Check sheet for the modelled part. Datum: model origin and axes. Units: mm. A direction names the side the tool comes from. Round coordinates to 2 decimals unless told otherwise and drop trailing zeros. Write each loop counter-clockwise with the first axis right and the second up, starting at its lowest first coordinate (ties: lowest second). Pieces come first, ordered by that corner, then holes.
Autodesk Inventor part; units mm, degrees
ref_plane "YZ Plane" through (0, 0, 0) normal (1, 0, 0) x (0, 1, 0)
ref_plane "XZ Plane" through (0, 0, 0) normal (0, 1, 0) x (-1, 0, 0)
ref_plane "XY Plane" through (0, 0, 0) normal (0, 0, 1) x (1, 0, 0)
sketch "スケッチ1" plane through (0, 0, 0) normal (0, 0, 1) x (1, 0, 0)
  line L0 (-120.5, 11.775) -> (120.5, 11.775) construction
  line L1 (120.5, 11.775) -> (120.5, -11.775) construction
  line L2 (120.5, -11.775) -> (-120.5, -11.775) construction
  line L3 (-120.5, -11.775) -> (-120.5, 11.775) construction
  circle A0 centre (-120.5, -11.775) radius 2.25
  circle A1 centre (-120.5, 11.775) radius 2.25
  circle A2 centre (-36.5, -11.775) radius 2.25
  circle A3 centre (42.5, -11.775) radius 2.25
  circle A4 centre (120.5, -11.775) radius 2.25
  line L4 (-129.5, 22.275) -> (-129.5, -20.275) construction
  line L5 (-129.5, 22.275) -> (129.5, 22.275) construction
  line L6 (129.5, 22.275) -> (129.5, -20.275) construction
  line L7 (129.5, -20.275) -> (-129.5, -20.275) construction
  circle A5 centre (-42.5, 17.275) radius 2.25
  circle A6 centre (42.5, 17.275) radius 2.25
  circle A7 centre (120.5, 11.775) radius 2.25
  line L8 (-129.5, -20.275) -> (129.5, -20.275)
  line L9 (129.5, -20.275) -> (129.5, 27.275)
  line L10 (129.5, 27.275) -> (-129.5, 27.275)
  line L11 (-129.5, 27.275) -> (-129.5, -20.275)
  point P0 (0, 0)
  point P1 (-120.5, 0)
  point P2 (0, 11.775)
  dimension "d0" = 23.55
  dimension "d1" = 84
  dimension "d3" = 79
  dimension "d4" = 78
  dimension "d5" = 4.5
  dimension "d6" = 9
  dimension "d7" = 9
  dimension "d8" = 8.5
  dimension "d9" = 10.5
  dimension "d10" = 5.5
  dimension "d11" = 78.1937
  dimension "d12" = 78.1937
  dimension "d13" = 78
  dimension "d14" = 85
  dimension "d15" = 78
  dimension "d16" = 5
extrude "押し出し1" add sketch "スケッチ1" along normal blind 4
sketch "スケッチ2" plane through (0, 0, 0) normal (0, 0, -1) x (-1, 0, 0)
  line L0 (129.5, 22.275) -> (-129.5, 22.275) construction
  line L1 (-129.5, 22.275) -> (129.5, 22.275)
  line L2 (129.5, 22.275) -> (129.5, 27.275)
  line L3 (129.5, 27.275) -> (-129.5, 27.275)
  line L4 (-129.5, 27.275) -> (-129.5, 22.275)
  line L5 (-129.5, 27.275) -> (129.5, 27.275) construction
  point P0 (0, 0)
extrude "押し出し2" add sketch "スケッチ2" along normal blind 47.4
fillet "フィレット1" radius 4 2 edges at (-129.5, -20.275, 2) (129.5, -20.275, 2)
fillet "フィレット2" [suppressed]
fillet "フィレット3" radius 4 2 edges at (129.5, 27.275, -21.7) (-129.5, 27.275, -21.7)
properties part number "kpd_70_cover" material "アルミニウム 6061"
1. Sectioned sample at A-A, the plane x = 120.5. Enter the section's corners in (y, z) (3 decimals), plus the area to 3 significant figures.
2. Sectioned sample at D-D, the plane y = 2. Enter the section's corners in (x, z), plus the area to 3 significant figures.
3. Sectioned sample at C-C, the plane z = -7. Enter the section's corners in (x, y) (3 decimals).
4. Go/stop test with flat-tipped pins: pin 1 (7 mm diameter, centred on x = 120.5, y = 11.775, fed in from +Z); pin 2 (2.5 mm diameter, centred on x = -120.5, y = 11.775, fed in from +Z); pin 3 (5 mm diameter, centred on x = -42.5, y = 17.275, fed in from -Z); pin 4 (2 mm diameter, centred on x = -38.5, z = -42, fed in from -Y) (3 decimals). Record where each tip stops, or that it passes through.
5. Release check for a two-part mould opening along Y. For faces 3 (the cylindrical face through (-118.422, 12.637, 1.972)), 4 (the flat face through (2, 27.275, -22)), 5 (the flat face through (-129.5, 9, 1)), 6 (the cylindrical face through (-44.748, 17.176, 1.972)) record: released by +Y, released by -Y, zero draft, split by the parting line, or undercut.
6. Sectioned sample at B-B, the plane x = -36.5. Enter the section's corners in (y, z) (3 decimals).
7. Set-up check for faces 1 (the flat face through (-2, 1, 0)), 2 (the cylindrical face through (122.646, -12.451, 1.972)): record each of +Z, -Z, +X, -X, +Y, -Y from which the full face is reachable in a straight line by a thin tool's end or side.
8. Scan lines: line 1 along Y through (x, z) = (-120.5, 2.3) (3 decimals); line 2 along Y through (x, z) = (-42.5, 2.9) (3 decimals); line 3 along Z through (x, y) = (-15, -10.5). Record each from-to range of solid material in increasing order.
Computed values:
1. outline: (-20.275, 0) - (-14.025, 0) - (-14.025, 4) - (-20.275, 4) - close; (-9.525, 0) - (9.525, 0) - (9.525, 4) - (-9.525, 4) - close; (14.025, 0) - (22.275, 0) - (22.275, -47.4) - (27.275, -47.4) - (27.275, 4) - (14.025, 4) - close
1. area: 391 mm2
2. outline: (-129.5, 0) - (129.5, 0) - (129.5, 4) - (-129.5, 4) - close
2. area: 1,040 mm2
3. outline: (-129.5, 22.275) - (129.5, 22.275) - (129.5, 23.275) arc R4 ccw to (125.5, 27.275) - (-125.5, 27.275) arc R4 ccw to (-129.5, 23.275) - close
4. pin 1: stops at z = 4
4. pin 2: passes through
4. pin 3: stops at z = 0
4. pin 4: stops at y = 22.275
5. face 3: undercut
5. face 4: released by +Y
5. face 5: zero draft
5. face 6: undercut
6. outline: (-20.275, 0) - (-14.025, 0) - (-14.025, 4) - (-20.275, 4) - close; (-9.525, 0) - (22.275, 0) - (22.275, -47.4) - (27.275, -47.4) - (27.275, 4) - (-9.525, 4) - close
7. face 1: -Z, +X, -X, -Y
7. face 2: +Z, -Z
8. line 1: y = -20.275 to -14.025, -9.525 to 9.525, 14.025 to 27.275
8. line 2: y = -20.275 to 15.025, 19.525 to 27.275
8. line 3: z = 0 to 4
